```python
from build123d import *

# Parameters (mm, degrees)
CROQUIS1_R              = 2
SALIENTE_EXTRUIR2_DEPTH = 1
CORTAR_EXTRUIR2_REACH   = 3


with BuildPart() as part:
    # Croquis1 → Saliente-Extruir2 (new body)
    with BuildSketch(Plane(origin=(0, 0, 0), x_dir=(1, 0, 0), z_dir=(0, 1, 0))):
        with BuildLine():
            Line((40.8, 27.5), (40.8, -27.5))
            ThreePointArc((40.8, -27.5), (40.067766953, -29.267766953), (38.3, -30))
            Line((38.3, -30), (-38.3, -30))
            ThreePointArc((-38.3, -30), (-40.067766953, -29.267766953), (-40.8, -27.5))
            Line((-40.8, -27.5), (-40.8, 27.5))
            ThreePointArc((-40.8, 27.5), (-40.067766953, 29.267766953), (-38.3, 30))
            Line((-38.3, 30), (38.3, 30))
            ThreePointArc((38.3, 30), (40.067766953, 29.267766953), (40.8, 27.5))
        make_face()
        with Locations((28.5, -24.8)):
            Circle(CROQUIS1_R, mode=Mode.SUBTRACT)
        with Locations((28.5, 24.8)):
            Circle(CROQUIS1_R, mode=Mode.SUBTRACT)
        with Locations((-28.5, 24.8)):
            Circle(CROQUIS1_R, mode=Mode.SUBTRACT)
        with Locations((-28.5, -24.8)):
            Circle(CROQUIS1_R, mode=Mode.SUBTRACT)
    extrude(amount=SALIENTE_EXTRUIR2_DEPTH)

    # Croquis2 → Cortar-Extruir2 (cut, up to next)
    with BuildSketch(Plane(origin=(0, 0, 0), x_dir=(1, 0, 0), z_dir=(0, 1, 0)), mode=Mode.PRIVATE) as cortar_extruir2_sk1:
        Polygon((-28.5, 17), (28.5, 17), (28.5, -17), (-28.5, -17), (-28.5, -4), align=None)
    cortar_extruir2_tool1 = extrude(cortar_extruir2_sk1.sketch, amount=CORTAR_EXTRUIR2_REACH, mode=Mode.PRIVATE) & part.part
    add(cortar_extruir2_tool1.solids().sort_by_distance((0, 0, 0))[0], mode=Mode.SUBTRACT)


solid = part.part
```
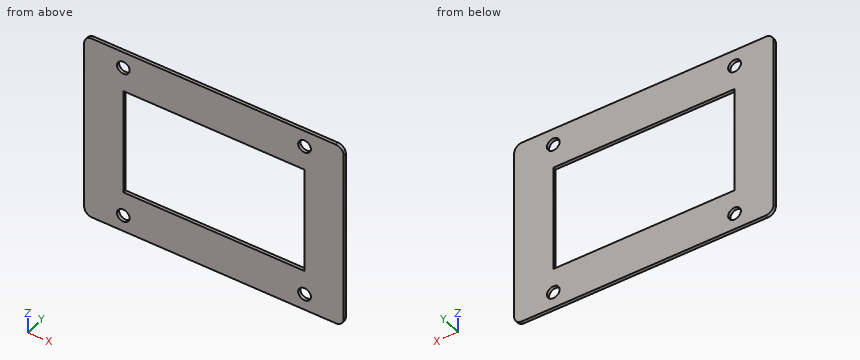
Design review of the part built by this model. Coordinates are the model's own, in mm. Coordinates: 2 decimals unless noted, no trailing zeros. Order: outer loops, then holes, each group sorted by start corner. A loop starts at its lowest first (then second) coordinate and runs counter-clockwise, first axis right, second up.
1) Take a section at A-A, the plane z = -15.5. Give the boundary of the cut face in (x, y).
2) Take a section at C-C, the plane y = 0.65. Give the boundary of the cut face in (x, z).
3) Take a section at B-B, the plane x = -24. Give the boundary of the cut face in (y, z).
4) Wall thickness on line 1 along X through (y, z) = (0.4, -24.8); line 2 along X through (y, z) = (0.75, -3); line 3 along Z through (x, y) = (25, 0.25): over which ranges is each line inside the solid? List them lowest first.
5) Clearance check with a flat-ended pin moving along its axis: pin 1 (3 mm diameter, centred on x = -28.5, z = -24.8, fed in from -Y). State where the tip first meets the part, or that it passes through.
6) Take a section at D-D, the plane z = 24.8. Give the boundary of the cut face in (x, y), and give its area (3 significant figures).
Returned:
1. outline: (-40.8, 0) - (-28.5, 0) - (-28.5, 1) - (-40.8, 1) - close; (28.5, 0) - (40.8, 0) - (40.8, 1) - (28.5, 1) - close
2. outline: (-40.8, -27.5) arc R2.5 ccw to (-38.3, -30) - (38.3, -30) arc R2.5 ccw to (40.8, -27.5) - (40.8, 27.5) arc R2.5 ccw to (38.3, 30) - (-38.3, 30) arc R2.5 ccw to (-40.8, 27.5) - close; hole circle Ø4 at (-28.5, -24.8); hole circle Ø4 at (-28.5, 24.8); hole (-28.5, -17) - (28.5, -17) - (28.5, 17) - (-28.5, 17) - close; hole circle Ø4 at (28.5, -24.8); hole circle Ø4 at (28.5, 24.8)
3. outline: (0, -30) - (1, -30) - (1, -17) - (0, -17) - close; (0, 17) - (1, 17) - (1, 30) - (0, 30) - close
4. line 1: x = -40.8 to -30.5, -26.5 to 26.5, 30.5 to 40.8
4. line 2: x = -40.8 to -28.5, 28.5 to 40.8
4. line 3: z = -30 to -17, 17 to 30
5. pin 1: passes through
6. outline: (-40.8, 0) - (-30.5, 0) - (-30.5, 1) - (-40.8, 1) - close; (-26.5, 0) - (26.5, 0) - (26.5, 1) - (-26.5, 1) - close; (30.5, 0) - (40.8, 0) - (40.8, 1) - (30.5, 1) - close
6. area: 73.6 mm2
